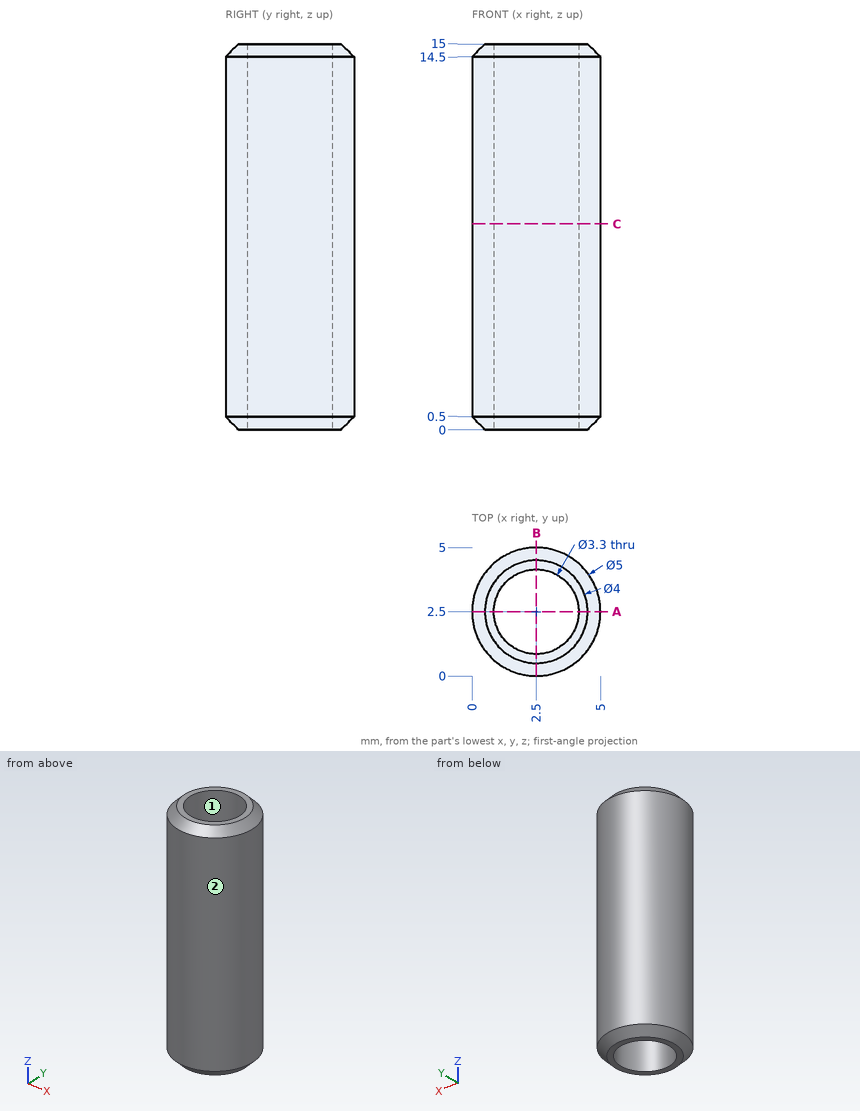
Answer from the drawing. Dimensions are ordinates in mm from the lowest x, y and z of the part. Give positions to 0.01 mm unless a question says otherwise; leave off trailing zeros. Order: outer loops, then holes, each group sorted by start corner. A loop starts at its lowest first (then second) coordinate and runs counter-clockwise, first axis right, second up.
(1) For a pull along X with two mould halves and no side action, classify the marked faces 1 and 2 as released by +X, released by -X, zero draft, split by the parting line, or undercut.
(2) Straight lines are drawn through the part: L1, parallel to Y at x = 2.5, z = 7; L2, parallel to Y at x = 3.65, z = 11.5. For each, find the intervals that lie inside material, in ascending order.
(3) Find section A-A (y = 2.5). Give the vertices of the cut face in (x, z).
(4) Find section C-C (z = 8). Give the vertices of the cut face in (x, y).
(5) Given pin 1 (2 mm diameter, centred on x = 1, y = 4, fed in from -Z); pin 2 (2 mm diameter, centred on y = 0.5, z = 4, fed in from -X), each flat-ended and moving along its own axis, determine where each tip first touches the part or whether it passes through.
Result sheet:
1. face 1: undercut
1. face 2: split by the parting line
2. L1: y = 0 to 0.85, 4.15 to 5
2. L2: y = 0.28 to 1.32, 3.68 to 4.72
3. outline: (0, 0.5) - (0.5, 0) - (0.85, 0) - (0.85, 15) - (0.5, 15) - (0, 14.5) - close; (4.15, 0) - (4.5, 0) - (5, 0.5) - (5, 14.5) - (4.5, 15) - (4.15, 15) - close
4. outline: circle Ø5 at (2.5, 2.5); hole circle Ø3.3 at (2.5, 2.5)
5. pin 1: stops at z = 0
5. pin 2: stops at x = 0.21
